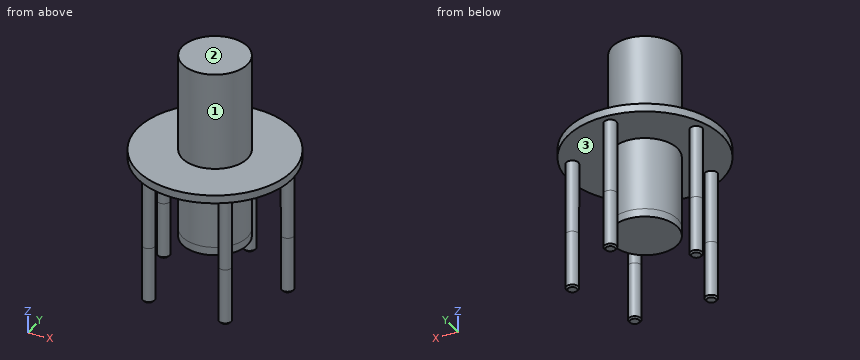
from build123d import *

# Parameters (mm, degrees)
SKETCH2_R             = 25.4
BOSS_EXTRUDE1_DEPTH   = 57.15
SKETCH2_R_2           = 4.7625
BOSS_EXTRUDE1_2_DEPTH = 57.15
BOSS_EXTRUDE1_3_DEPTH = 57.15
BOSS_EXTRUDE1_4_DEPTH = 57.15
BOSS_EXTRUDE1_5_DEPTH = 57.15
BOSS_EXTRUDE1_6_DEPTH = 57.15
SKETCH3_R             = 60.325
BOSS_EXTRUDE2_DEPTH   = 6.35
SKETCH4_R             = 25.4
BOSS_EXTRUDE3_DEPTH   = 6.35
SKETCH5_R             = 4.7625
BOSS_EXTRUDE4_DEPTH   = 44.45
CHAMFER1_SIZE         = 1.27
SKETCH7_R             = 25.4
BOSS_EXTRUDE5_DEPTH   = 76.2


with BuildPart() as part:
    # Sketch2 → Boss-Extrude1 (new body)
    with BuildSketch(Plane.XY):
        with Locations((-60.561942489, 11.211112057)):
            Circle(SKETCH2_R)
    extrude(amount=BOSS_EXTRUDE1_DEPTH)



with BuildPart() as body_2:
    # Sketch2 → Boss-Extrude1 2 (new body)
    with BuildSketch(Plane.XY):
        with Locations((-12.248271462, 26.909175371)):
            Circle(SKETCH2_R_2)
    extrude(amount=BOSS_EXTRUDE1_2_DEPTH)


with BuildPart() as body_3:
    # Sketch2 → Boss-Extrude1 3 (new body)
    with BuildSketch(Plane.XY):
        with Locations((-60.561942489, 62.011112057)):
            Circle(SKETCH2_R_2)
    extrude(amount=BOSS_EXTRUDE1_3_DEPTH)


with BuildPart() as body_4:
    # Sketch2 → Boss-Extrude1 4 (new body)
    with BuildSketch(Plane.XY):
        with Locations((-108.875613517, 26.909175371)):
            Circle(SKETCH2_R_2)
    extrude(amount=BOSS_EXTRUDE1_4_DEPTH)


with BuildPart() as body_5:
    # Sketch2 → Boss-Extrude1 5 (new body)
    with BuildSketch(Plane.XY):
        with Locations((-90.421433306, -29.886951258)):
            Circle(SKETCH2_R_2)
    extrude(amount=BOSS_EXTRUDE1_5_DEPTH)


with BuildPart() as body_6:
    # Sketch2 → Boss-Extrude1 6 (new body)
    with BuildSketch(Plane.XY):
        with Locations((-30.702451673, -29.886951258)):
            Circle(SKETCH2_R_2)
    extrude(amount=BOSS_EXTRUDE1_6_DEPTH)


with BuildPart() as part_1:
    add(part.part)

    add(body_2.part)  # Boss-Extrude2 merges body 2

    add(body_3.part)  # Boss-Extrude2 merges body 3

    add(body_4.part)  # Boss-Extrude2 merges body 4

    add(body_5.part)  # Boss-Extrude2 merges body 5

    add(body_6.part)  # Boss-Extrude2 merges body 6
    # Sketch3 → Boss-Extrude2 (add)
    with BuildSketch(Plane.XY.offset(57.15)):
        with Locations((-60.561942489, 11.211112057)):
            Circle(SKETCH3_R)
    extrude(amount=BOSS_EXTRUDE2_DEPTH)

    # Sketch4 → Boss-Extrude3 (add)
    with BuildSketch(Plane(origin=(0, 0, 0), x_dir=(-1, 0, 0), z_dir=(0, 0, -1))):
        with Locations((60.561942489, 11.211112057)):
            Circle(SKETCH4_R)
    extrude(amount=BOSS_EXTRUDE3_DEPTH)

    # Sketch5 → Boss-Extrude4 (add)
    with BuildSketch(Plane(origin=(0, 0, 0), x_dir=(-1, 0, 0), z_dir=(0, 0, -1))):
        with Locations((12.248271462, 26.909175371)):
            Circle(SKETCH5_R)
        with Locations((30.702451673, -29.886951258)):
            Circle(SKETCH5_R)
        with Locations((90.421433306, -29.886951258)):
            Circle(SKETCH5_R)
        with Locations((108.875613517, 26.909175371)):
            Circle(SKETCH5_R)
        with Locations((60.561942489, 62.011112057)):
            Circle(SKETCH5_R)
    extrude(amount=BOSS_EXTRUDE4_DEPTH)

    # Chamfer1
    chamfer1_edges = [part_1.edges().sort_by_distance(p)[0] for p in [
        (-7.485771462, 26.909175371, -44.45),
        (-25.939951673, -29.886951258, -44.45),
        (-85.658933306, -29.886951258, -44.45),
        (-104.113113517, 26.909175371, -44.45),
        (-55.799442489, 62.011112057, -44.45),
    ]]
    chamfer(chamfer1_edges, length=CHAMFER1_SIZE)

    # Sketch7 → Boss-Extrude5 (add)
    with BuildSketch(Plane.XY.offset(63.5)):
        with Locations((-60.561942489, 11.211112057)):
            Circle(SKETCH7_R)
    extrude(amount=BOSS_EXTRUDE5_DEPTH)


solid = part_1.part
Geometry check sheet. Reference: the model listing, model coordinates, mm. Face numbers are marked on the shaded views. A direction names the side the tool comes from. Round coordinates to 2 decimals unless told otherwise and drop trailing zeros. Order: outer loops, then holes, each group sorted by start corner. A loop starts at its lowest first (then second) coordinate and runs counter-clockwise, first axis right, second up. Notation, with made-up numbers: M 71,2 L 120,2 A19 ccw 120,16 Z; hole C 82,24.5 d8. An arc over 180 degrees is marked long. Answer in a Markdown table with one row per item. Add a question column.
Item 1: Sectioned sample at D-D, the plane z = 97. Enter the section's corners in (x, y), plus the area to 3 significant figures.
Item 2: Set-up check for the marked faces 1, 2 and 3: record each of +Z, -Z, +X, -X, +Y, -Y from which the full face is reachable in a straight line by a thin tool's end or side.
Item 3: Sectioned sample at C-C, the plane y = -3. Enter the section's corners in (x, z), plus the area to 3 significant figures.
Item 4: Material ranges on L1, parallel to Z at x = -52.5, y = -14.5; L2, parallel to X at y = -34, z = -19; L3, parallel to X at y = 15, z = 44, recorded low to high. Write a range as [from, to].
Item 5: Depth check by flat-ended pin: pin 1 Ø3 at (x, y) = (-90, -13) entering from +Z; pin 2 Ø4 at (x, z) = (-62, -16) entering from -Y; pin 3 Ø12 at (y, z) = (-11, -11.5) entering from -X; pin 4 Ø1.5 at (y, z) = (56, 9) entering from -X. Enter the tip coordinate at first touch or a pass-through.
Item 6: Sectioned sample at B-B, the plane x = -71. Enter the section's corners in (y, z), plus the area to 3 significant figures.
Item 7: Sectioned sample at A-A, the plane z = 24.5. Enter the section's corners in (x, y) (1 decimal).
Filled in:
| question | item | result |
|---|---|---|
| 1 | outline | C -60.56,11.21 d50.8 |
| 1 | area | 2,030 mm² |
| 2 | face 1 | +Z |
| 2 | face 2 | +Z, +X, -X, +Y, -Y |
| 2 | face 3 | -Z |
| 3 | outline | M -119.19,57.15 L -81.61,57.15 L -81.61,-6.35 L -39.51,-6.35 L -39.51,57.15 L -1.93,57.15 L -1.93,63.5 L -39.51,63.5 L -39.51,139.7 L -81.61,139.7 L -81.61,63.5 L -119.19,63.5 Z |
| 3 | area | 6,630 mm² |
| 4 | L1 | z = [57.15, 63.5] |
| 4 | L2 | x = [-92.82, -88.02], [-33.1, -28.3] |
| 4 | L3 | x = [-85.68, -35.45] |
| 5 | pin 1 | stops at z = 63.5 |
| 5 | pin 2 | stops at y = 57.25 |
| 5 | pin 3 | stops at x = -77.27 |
| 5 | pin 4 | passes through |
| 6 | outline | M -48.2,57.15 L -11.95,57.15 L -11.95,-6.35 L 34.37,-6.35 L 34.37,57.15 L 70.63,57.15 L 70.63,63.5 L 34.37,63.5 L 34.37,139.7 L -11.95,139.7 L -11.95,63.5 L -48.2,63.5 Z |
| 6 | area | 7,220 mm² |
| 7 | outline | C -108.9,26.9 d9.5; C -90.4,-29.9 d9.5; C -60.6,11.2 d50.8; C -60.6,62 d9.5; C -30.7,-29.9 d9.5; C -12.2,26.9 d9.5 |
